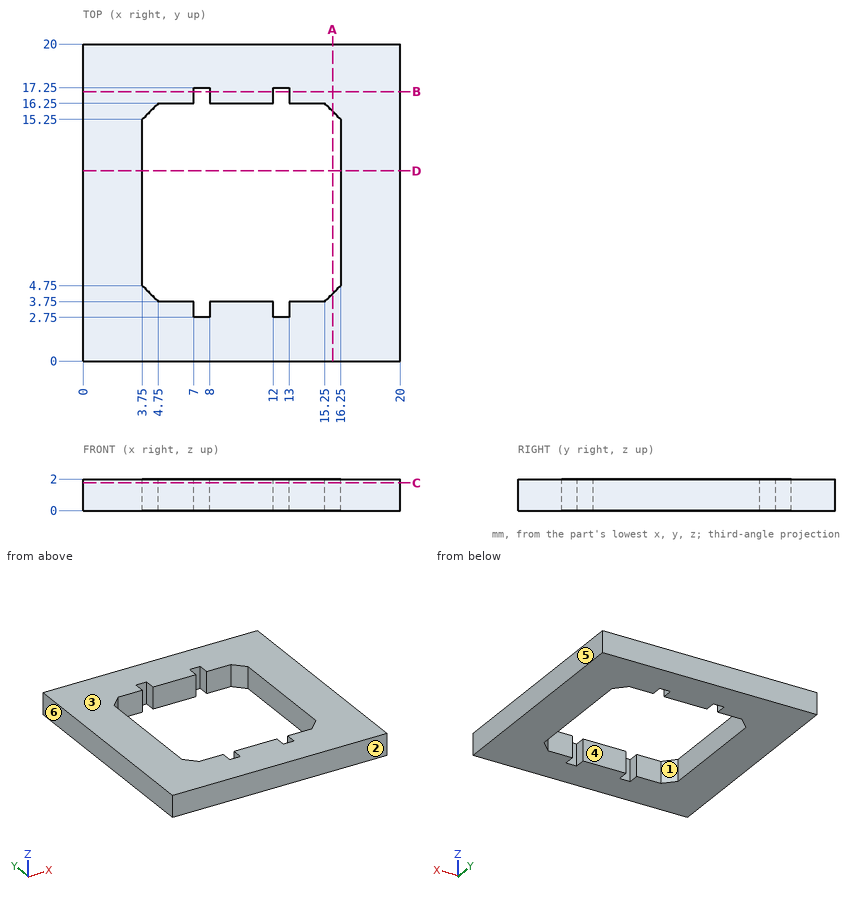
Verification items for this drawing (mm, ordinates from the low corner). A direction names the side the tool comes from. Give positions to 0.01 mm unless a question says otherwise; leave off trailing zeros. Write each loop counter-clockwise with the first axis right and the second up, starting at its lowest first coordinate (ties: lowest second). Pieces come first, ordered by that corner, then holes.
1) Gauge pin test, flat end, axial feed: pin 1 (8 mm diameter, centred on x = 6, y = 6.5, fed in from +Z). Record the tip position at first contact, or that the pin passes through.
2) Material ranges on L1, parallel to X at y = 16.5, z = 1.55; L2, parallel to X at y = 14.25, z = 1.45, recorded low to high.
3) Section check D-D, the plane y = 12. Record the boundary of the cut face in (x, z).
4) Section check C-C, the plane z = 1.75. Record the boundary of the cut face in (x, y), and give its area (3 significant figures).
5) Section check B-B, the plane y = 17. Record the boundary of the cut face in (x, z), and give its area (3 significant figures).
6) Section check A-A, the plane x = 15.75. Record the boundary of the cut face in (y, z).
7) Access from +Z, -Z, +X, -X, +Y, -Y to the whole of each face (thin tool, end or side, straight path). Record for the marked faces 1 and 2.
8) Release check for a two-part mould opening along X. For the marked faces 3, 4, 5 and 6 record: pulls with the +X half, pulls with the -X half, needs draft (parallel to the pull), parting line crosses it, or undercut.
Computed:
1. pin 1: stops at z = 2
2. L1: x = 0 to 7, 8 to 12, 13 to 20
2. L2: x = 0 to 3.75, 16.25 to 20
3. outline: (0, 0) - (3.75, 0) - (3.75, 2) - (0, 2) - close; (16.25, 0) - (20, 0) - (20, 2) - (16.25, 2) - close
4. outline: (0, 0) - (20, 0) - (20, 20) - (0, 20) - close; hole (3.75, 4.75) - (4.75, 3.75) - (7, 3.75) - (7, 2.75) - (8, 2.75) - (8, 3.75) - (12, 3.75) - (12, 2.75) - (13, 2.75) - (13, 3.75) - (15.25, 3.75) - (16.25, 4.75) - (16.25, 15.25) - (15.25, 16.25) - (13, 16.25) - (13, 17.25) - (12, 17.25) - (12, 16.25) - (8, 16.25) - (8, 17.25) - (7, 17.25) - (7, 16.25) - (4.75, 16.25) - (3.75, 15.25) - close
4. area: 242 mm2
5. outline: (0, 0) - (7, 0) - (7, 2) - (0, 2) - close; (8, 0) - (12, 0) - (12, 2) - (8, 2) - close; (13, 0) - (20, 0) - (20, 2) - (13, 2) - close
5. area: 36.0 mm2
6. outline: (0, 0) - (4.25, 0) - (4.25, 2) - (0, 2) - close; (15.75, 0) - (20, 0) - (20, 2) - (15.75, 2) - close
7. face 1: +Z, -Z
7. face 2: +Z, -Z, +X, -X, -Y
8. face 3: needs draft
8. face 4: undercut
8. face 5: pulls with the +X half
8. face 6: pulls with the -X half
